Design review of the part built by this model. Coordinates are the model's own, in mm. Face numbers are marked on the shaded views. Give positions to 0.01 mm unless a question says otherwise; leave off trailing zeros. Write each loop counter-clockwise with the first axis right and the second up, starting at its lowest first coordinate (ties: lowest second). Pieces come first, ordered by that corner, then holes.
```python
from build123d import *

# Parameters (mm, degrees)
ESQUISSE1_R                                = 84.1225
BOSS_EXTRU_1_DEPTH                         = 5.75
ESQUISSE2_R                                = 53.13
BOSS_EXTRU_2_DEPTH                         = 5.75
TROU_TARAUD_M31_D                          = 2.5
TROU_TARAUD_M31_DEPTH                      = 12.5
TROU_TARAUD_M31_TIP                        = 0.751075774
CHAMBRAGE_POUR_VIS_T_TE_HEXAGONALE_2_COUNT = 2
CHAMBRAGE_POUR_VIS_T_TE_HEXAGONALE_2_PITCH = 46.9428037
CHAMBRAGE_POUR_VIS_T_TE_HEXAGONALE_3_COUNT = 2
CHAMBRAGE_POUR_VIS_T_TE_HEXAGONALE_3_PITCH = 118.863351538
CHAMBRAGE_POUR_VIS_T_TE_HEXAGONALE_4_COUNT = 2
CHAMBRAGE_POUR_VIS_T_TE_HEXAGONALE_4_PITCH = 135.166416173
CHAMBRAGE_POUR_VIS_T_TE_HEXAGONALE_5_COUNT = 2
CHAMBRAGE_POUR_VIS_T_TE_HEXAGONALE_5_PITCH = 118.863351538
CHAMBRAGE_POUR_VIS_T_TE_HEXAGONALE_6_COUNT = 2
CHAMBRAGE_POUR_VIS_T_TE_HEXAGONALE_6_PITCH = 88.223612472


with BuildPart() as part:
    # Esquisse1 → Boss.-Extru.1 (new body)
    with BuildSketch(Plane(origin=(0, 0, 0), x_dir=(1, 0, 0), z_dir=(0, 1, 0))):
        Circle(ESQUISSE1_R)
    extrude(amount=-BOSS_EXTRU_1_DEPTH)

    # Esquisse2 → Boss.-Extru.2 (add)
    with BuildSketch(Plane(origin=(0, 0, 0), x_dir=(1, 0, 0), z_dir=(0, 1, 0))):
        Circle(ESQUISSE2_R)
    extrude(amount=BOSS_EXTRU_2_DEPTH)

    # Trou taraudé M31
    with Locations(Plane(origin=(0, -5.75, -50), x_dir=(0, 0, -1), z_dir=(0, -1, 0))):
        with Locations((0, 0), (-50, -50), (-100, 0), (-50, 50)):
            Hole(TROU_TARAUD_M31_D / 2, depth=TROU_TARAUD_M31_DEPTH)
            with Locations((0, 0, -(TROU_TARAUD_M31_DEPTH + TROU_TARAUD_M31_TIP / 2))):  # 118° drill point
                Cone(0, TROU_TARAUD_M31_D / 2, TROU_TARAUD_M31_TIP, mode=Mode.SUBTRACT)

    # Esquisse7 → Chambrage pour vis à tête hexagonale M31 (revolve, cut)
    with BuildSketch(Plane(origin=(-26.582568127, -5.75, 63.268205691), x_dir=(0, 0, -1), z_dir=(1, 0, 0))):
        Polygon((0, 0), (0, 11.5), (1.7, 11.5), (1.7, 2), (4.6755, 2), (4.6755, 0.025), (4.7005, 0), align=None)
    chambrage_pour_vis_t_te_hexagonale_m31 = revolve(axis=Axis((-26.582568127, -12.1, 63.268205691), (0, 1, 0)), mode=Mode.SUBTRACT)

    # Chambrage pour vis _ t_te hexagonale 2: Chambrage pour vis à tête hexagonale M31 ×2
    with Locations(*[Vector(0.998814611, 0, 0.048676196) * (i * CHAMBRAGE_POUR_VIS_T_TE_HEXAGONALE_2_PITCH) for i in range(1, CHAMBRAGE_POUR_VIS_T_TE_HEXAGONALE_2_COUNT)]):
        add(chambrage_pour_vis_t_te_hexagonale_m31, mode=Mode.SUBTRACT)

    # Chambrage pour vis _ t_te hexagonale 3: Chambrage pour vis à tête hexagonale M31 ×2
    with Locations(*[Vector(0.796424839, 0, -0.604737527) * (i * CHAMBRAGE_POUR_VIS_T_TE_HEXAGONALE_3_PITCH) for i in range(1, CHAMBRAGE_POUR_VIS_T_TE_HEXAGONALE_3_COUNT)]):
        add(chambrage_pour_vis_t_te_hexagonale_m31, mode=Mode.SUBTRACT)

    # Chambrage pour vis _ t_te hexagonale 4: Chambrage pour vis à tête hexagonale M31 ×2
    with Locations(*[Vector(0.541562128, 0, -0.840660729) * (i * CHAMBRAGE_POUR_VIS_T_TE_HEXAGONALE_4_PITCH) for i in range(1, CHAMBRAGE_POUR_VIS_T_TE_HEXAGONALE_4_COUNT)]):
        add(chambrage_pour_vis_t_te_hexagonale_m31, mode=Mode.SUBTRACT)

    # Chambrage pour vis _ t_te hexagonale 5: Chambrage pour vis à tête hexagonale M31 ×2
    with Locations(*[Vector(-0.125505642, 0, -0.992092906) * (i * CHAMBRAGE_POUR_VIS_T_TE_HEXAGONALE_5_PITCH) for i in range(1, CHAMBRAGE_POUR_VIS_T_TE_HEXAGONALE_5_COUNT)]):
        add(chambrage_pour_vis_t_te_hexagonale_m31, mode=Mode.SUBTRACT)

    # Chambrage pour vis _ t_te hexagonale 6: Chambrage pour vis à tête hexagonale M31 ×2
    with Locations(*[Vector(-0.457252483, 0, -0.889336925) * (i * CHAMBRAGE_POUR_VIS_T_TE_HEXAGONALE_6_PITCH) for i in range(1, CHAMBRAGE_POUR_VIS_T_TE_HEXAGONALE_6_COUNT)]):
        add(chambrage_pour_vis_t_te_hexagonale_m31, mode=Mode.SUBTRACT)


solid = part.part
```
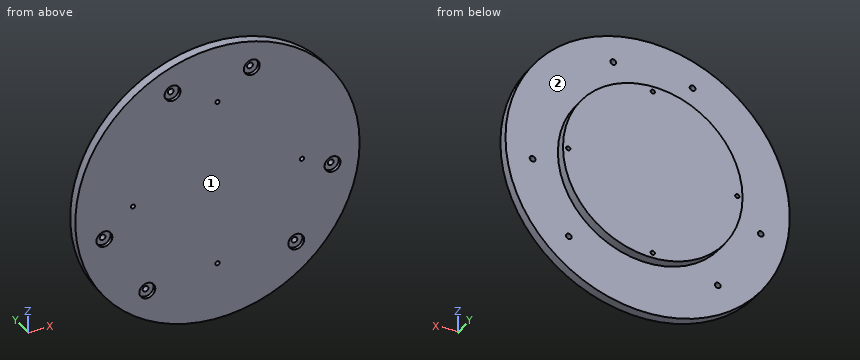
(1) Mouldability with a two-part tool opening along Y and no side actions: class the marked faces 1 and 2 as pulls with the +Y half, pulls with the -Y half, needs draft (parallel to the pull), parting line crosses it, or undercut.
Resolved:
face 1: pulls with the -Y half
face 2: pulls with the +Y half
(2) To check wall thickness, follow L1, parallel to Y at x = 77, z = 27.5; L2, parallel to X at y = -2, z = -2.5; L3, parallel to Z at x = 21, y = -0.75. State the ranges of each line that lie inside material, in increasing order.
Resolved:
L1: y = -5.75 to 0
L2: x = -84.09 to 84.09
L3: z = -81.46 to 64, 67.1 to 81.46
(3) Consider section B-B, the plane z = 35. Give the boundary of the cut face in (x, y).
Resolved:
outline: (-76.5, -5.75) - (76.5, -5.75) - (76.5, 0) - (39.97, 0) - (39.97, 5.75) - (-39.97, 5.75) - (-39.97, 0) - (-76.5, 0) - close
(4) Clearance check with flat-ended pins moving along their axes: P1, Ø8.5, axis at x = 20.3, z = 65.55, coming from the -Y side; P2, Ø1, axis at y = -3.5, z = 19, coming from the -X side; P3, Ø6, axis at x = 47.5, y = 2.5, coming from the +Z side. State where each tip first meets the part, or that it passes through.
Resolved:
P1: stops at y = -3.75
P2: stops at x = -82.06
P3: stops at z = 70.53
(5) Consider section A-A, the plane y = 4. Give the boundary of the cut face in (x, z).
Resolved:
outline: circle Ø106.26 at (0, 0); hole circle Ø2.5 at (-50, 0); hole circle Ø2.5 at (0, -50); hole circle Ø2.5 at (0, 50); hole circle Ø2.5 at (50, 0)
(6) Consider section C-C, the plane x = 36.5. Give the boundary of the cut face in (y, z).
Resolved:
outline: (-5.75, -75.79) - (0, -75.79) - (0, -38.61) - (5.75, -38.61) - (5.75, 38.61) - (0, 38.61) - (0, 75.79) - (-5.75, 75.79) - close
